The listing builds one solid part. Answer for the finished solid, in the listing's coordinates (mm). Give positions to 0.01 mm unless a question says otherwise; leave off trailing zeros. Write each loop counter-clockwise with the first axis right and the second up, starting at its lowest first coordinate (ties: lowest second). Pieces come first, ordered by that corner, then holes.
```python
from build123d import *

# Parameters (mm, degrees)
F0_W = 43.9448170364
F0_H = 40.1015970856
F3_R = 5.08
F5_D = 6.35


with BuildPart() as f2:
    # F2: sweep along a path in F1
    with BuildLine(Plane.XZ) as f2_path:
        Line((0, 0), (0, 20.9540724754))
    # F0 (on Top) → F2 (sweep)
    with BuildSketch(Plane.XY):
        with Locations((-5.7449191809, 4.2037246749)):
            Rectangle(F0_W, F0_H)
    sweep(path=f2_path.line)

    # F3
    f3_edges = [f2.edges().sort_by_distance(p)[0] for p in [
        (-27.717328, 4.203725, 20.954072),
        (16.227489, 4.203725, 20.954072),
        (-5.744919, 24.254523, 20.954072),
        (-5.744919, -15.847074, 20.954072),
        (16.227489, -15.847074, 10.477036),
        (-27.717328, -15.847074, 10.477036),
        (-27.717328, 24.254523, 10.477036),
        (16.227489, 24.254523, 10.477036),
        (-5.744919, 24.254523, 0),
        (-27.717328, 4.203725, 0),
        (-5.744919, -15.847074, 0),
        (16.227489, 4.203725, 0),
    ]]
    fillet(f3_edges, radius=F3_R)

    # F5 (through all)
    with Locations(Plane.XY.offset(20.9540724754)):
        with Locations((-5.5084819905, 4.9320813268)):
            Hole(F5_D / 2)


solid = f2.part
```
Item 1: Each of these flat-tipped pins is pushed along its axis until it touches: P1, Ø3, axis at y = 9, z = 2.5, coming from the +X side; P2, Ø5.5, axis at x = -5.51, y = 4.93, coming from the +Z side; P3, Ø3, axis at x = -20.5, z = 18.5, coming from the -Y side. Where does it stop, or does it pass through?
Conclusion:
P1: stops at x = 16.11
P2: passes through
P3: stops at y = -15.72
Item 2: Determine the mould class of faces 1 (the face through (14.779, 22.727, 10.553)), 2 (the face through (-5.1, 8.08, 10.33)), 3 (the face through (-5.51, -14.4, 1.53)) for opening direction X: pulls with the +X half, pulls with the -X half, needs draft (parallel to the pull), parting line crosses it, or undercut.
Conclusion:
face 1: pulls with the +X half
face 2: undercut
face 3: needs draft
Item 3: A cutting plane is placed at A-A, the plane z = 12. Give the vertices of the cut face in (x, y) (3 decimals).
Conclusion:
outline: (-27.717, -10.767) arc R5.08 ccw to (-22.637, -15.847) - (11.147, -15.847) arc R5.08 ccw to (16.227, -10.767) - (16.227, 19.175) arc R5.08 ccw to (11.147, 24.255) - (-22.637, 24.255) arc R5.08 ccw to (-27.717, 19.175) - close; hole circle Ø6.35 at (-5.508, 4.932)
Item 4: A cutting plane is placed at C-C, the plane x = -21.5. Give the vertices of the cut face in (y, z).
Conclusion:
outline: (-15.85, 5.08) arc R5.08 ccw to (-10.77, 0) - (19.17, 0) arc R5.08 ccw to (24.25, 5.08) - (24.25, 15.87) arc R5.08 ccw to (19.17, 20.95) - (-10.77, 20.95) arc R5.08 ccw to (-15.85, 15.87) - close
Item 5: Consider probe 1 along X at (y, z) = (5, 14.75); probe 2 along X at (y, z) = (2, 10); probe 3 along Y at (x, z) = (-8, 11.75). Determine where each line is inside the solid, lowest interval first.
Conclusion:
probe 1: x = -27.72 to -8.68, -2.33 to 16.23
probe 2: x = -27.72 to -6.73, -4.29 to 16.23
probe 3: y = -15.85 to 2.96, 6.9 to 24.25
Item 6: A cutting plane is placed at B-B, the plane y = 17.5. Give the vertices of the cut face in (x, z), plus the area to 3 significant figures.
Conclusion:
outline: (-27.72, 5.08) arc R5.08 ccw to (-22.64, 0) - (11.15, 0) arc R5.08 ccw to (16.23, 5.08) - (16.23, 15.87) arc R5.08 ccw to (11.15, 20.95) - (-22.64, 20.95) arc R5.08 ccw to (-27.72, 15.87) - close
area: 899 mm2
Item 7: A cutting plane is placed at D-D, the plane z = 3.25. Give the vertices of the cut face in (x, y) (3 decimals).
Conclusion:
outline: (-27.376, -10.767) arc R4.739 ccw to (-22.637, -15.506) - (11.147, -15.506) arc R4.739 ccw to (15.886, -10.767) - (15.886, 19.175) arc R4.739 ccw to (11.147, 23.913) - (-22.637, 23.913) arc R4.739 ccw to (-27.376, 19.175) - close; hole circle Ø6.35 at (-5.508, 4.932)
